Build history of the part. All positions in model axes, mm. A direction names the side the tool comes from. Round coordinates to 2 decimals unless told otherwise and drop trailing zeros. Order: outer loops, then holes, each group sorted by start corner. A loop starts at its lowest first (then second) coordinate and runs counter-clockwise, first axis right, second up. Notation, with made-up numbers: (-33, 28.5) -> (-6, 28.5) arc R8 ccw to (-6, 35.5) -> close; hole circle Ø8 at (47.5, 65.5). An arc over 180 degrees is marked (long way). Answer as a JSON object with one key per item and string values.
from build123d import *

# Parameters (mm, degrees)
SKETCH1_R           = 10
SKETCH1_W           = 30
SKETCH1_H           = 20
BOSS_EXTRUDE1_DEPTH = 15
BOSS_EXTRUDE2_DEPTH = 25
SKETCH3_R           = 5
CUT_EXTRUDE1_DEPTH  = 58
FILLET1_R           = 10


with BuildPart() as part:
    # Sketch1 → Boss-Extrude1 (new body)
    # profile 1 of 3: a face of its own
    with BuildSketch(Plane(origin=(0, 0, 0), x_dir=(1, 0, 0), z_dir=(0, 1, 0))):
        Polygon((-15, -39.607549464), (-24.990355032, -0.301923542), (-15, 39.00370238), (15, 39.00370238), (24.990355032, -0.301923542), (15, -39.607549464), align=None)
        with Locations(Location((0, 0, 0), (0, 0, 270))):
            Circle(SKETCH1_R, mode=Mode.SUBTRACT)
    # profile 2 of 3: a face of its own
    with BuildSketch(Plane(origin=(0, 0, 0), x_dir=(1, 0, 0), z_dir=(0, 1, 0))):
        with Locations((0, -49.607549464)):
            Rectangle(SKETCH1_W, SKETCH1_H)
    # profile 3 of 3: a face of its own
    with BuildSketch(Plane(origin=(0, 0, 0), x_dir=(1, 0, 0), z_dir=(0, 1, 0))):
        with Locations((0, 49.00370238)):
            Rectangle(SKETCH1_W, SKETCH1_H)
    extrude(amount=BOSS_EXTRUDE1_DEPTH)

    # Sketch2 → Boss-Extrude2 (add)
    with BuildSketch(Plane(origin=(0, 15, 0), x_dir=(1, 0, 0), z_dir=(0, 1, 0))):
        Polygon((15, 59.00370238), (5.264710161, 59.00370238), (5.264710161, 37.962238036), (15.264710161, 37.962238036), (15, 39.00370238), align=None)
        Polygon((-5, 59.00370238), (-15, 59.00370238), (-15, 39.00370238), (-15, 37.962238036), (-5, 37.962238036), align=None)
        Polygon((-5, -59.00370238), (-5, -37.962238036), (-15, -37.962238036), (-15, -39.607549464), (-15, -59.00370238), align=None)
        Polygon((15, -39.607549464), (15.264710161, -38.56608512), (15.264710161, -37.962238036), (5.264710161, -37.962238036), (5.264710161, -59.00370238), (15, -59.00370238), align=None)
    extrude(amount=BOSS_EXTRUDE2_DEPTH)

    # Sketch3 → Cut-Extrude1 (cut)
    with BuildSketch(Plane(origin=(15, 0, 0), x_dir=(0, 0, -1), z_dir=(1, 0, 0))):
        with Locations((-49.607549464, 30)):
            Circle(SKETCH3_R)
        with Locations((49.00370238, 30)):
            Circle(SKETCH3_R)
    extrude(amount=-CUT_EXTRUDE1_DEPTH, mode=Mode.SUBTRACT)

    # Fillet1
    fillet1_edges = [part.edges().sort_by_distance(p)[0] for p in [
        (10.13235508, 40, -59.00370238),
        (10.264710161, 40, -37.962238036),
        (-10, 40, -59.00370238),
        (-10, 40, -37.962238036),
        (10.264710161, 40, 37.962238036),
        (-10, 40, 37.962238036),
        (10.13235508, 40, 59.00370238),
        (-10, 40, 59.00370238),
    ]]
    fillet(fillet1_edges, radius=FILLET1_R)


solid = part.part
1) Cut at C-C, the plane z = 4. Give the cut face in (x, y), plus the area to 3 significant figures.
Checked values:
{"outline": "(-24.05, 0) -> (-9.17, 0) -> (-9.17, 15) -> (-24.05, 15) -> close; (9.17, 0) -> (24.05, 0) -> (24.05, 15) -> (9.17, 15) -> close", "area": "447 mm²"}
2) Which spindle directions (+Z, -Z, +X, -X, +Y, -Y) get a long thin tool onto all of the face, cutting with end or side? Do faces 4 (the face through (-20.065, 7.395, -19.076)), 5 (the face through (10, 22, -37.962)), 6 (the face through (-10, 22, 59.004)), 7 (the face through (10.2, 28.08, 44.99)), 8 (the face through (5.265, 24.5, -48.6)). Say none if no direction does.
Checked values:
{"face 4": "-Z, -X, +Y, -Y", "face 5": "+X, -X, +Y", "face 6": "+Z, +X, -X, +Y", "face 7": "+X, -X", "face 8": "+Z, -Z, +Y"}
3) Cut at A-A, the plane y = 10.5. Give the cut face in (x, z).
Checked values:
{"outline": "(-24.99, 0.3) -> (-15, -39) -> (-15, -59) -> (15, -59) -> (15, -39) -> (24.99, 0.3) -> (15, 39.61) -> (15, 59.61) -> (-15, 59.61) -> (-15, 39.61) -> close; hole circle Ø20 at (0, 0)"}
4) Cut at B-B, the plane x = -12.5. Give the cut face in (y, z).
Checked values:
{"outline": "(0, -59) -> (30, -59) arc R10 ccw to (40, -49) -> (40, -47.96) arc R10 ccw to (30, -37.96) -> (15, -37.96) -> (15, 37.96) -> (30, 37.96) arc R10 ccw to (40, 47.96) -> (40, 49) arc R10 ccw to (30, 59) -> (15, 59) -> (15, 59.61) -> (0, 59.61) -> close; hole circle Ø10 at (30, -49); hole circle Ø10 at (30, 49.61)"}
5) Cut at D-D, the plane z = -8.5. Give the cut face in (x, y).
Checked values:
{"outline": "(-22.75, 0) -> (-5.27, 0) -> (-5.27, 15) -> (-22.75, 15) -> close; (5.27, 0) -> (22.75, 0) -> (22.75, 15) -> (5.27, 15) -> close"}
6) Probe L1, parallel to X at y = 22, z = 52; L2, parallel to Y at x = 5, z = 15; L3, parallel to Z at x = -6.5, y = 26. List the from-to ranges inside material, lowest first. Write a range as from..to.
Checked values:
{"L1": "x = -15..-5, 5.26..15", "L2": "y = 0..15", "L3": "z = -59..-52, -46..-37.96, 37.96..46.61, 52.61..59"}
7) Pull direction Y, two halves, no side cores. Call faces 1 (the face through (10.064, 36.993, -56.152)), 2 (the face through (15, 20, 50)), 3 (the face through (-9.93, 26.958, -45.036)): pulls with the +Y half, pulls with the -Y half, needs draft (parallel to the pull), parting line crosses it, or undercut.
Checked values:
{"face 1": "pulls with the +Y half", "face 2": "needs draft", "face 3": "undercut"}
8) Flat gauge pins, fed straight in: pin 1 Ø3 at (y, z) = (16, -47) entering from -X; pin 2 Ø8 at (x, y) = (11, 22) entering from +Z; pin 3 Ø16 at (x, z) = (0, 0) entering from -Y; pin 4 Ø8 at (x, z) = (0, 10.5) entering from +Y. Where does each tip first touch, or does it go through?
Checked values:
{"pin 1": "stops at x = -15", "pin 2": "stops at z = 59", "pin 3": "passes through", "pin 4": "stops at y = 15"}
